Work out the finished part from the listing and answer in its coordinate system (mm). A direction names the side the tool comes from. Round coordinates to 2 decimals unless told otherwise and drop trailing zeros. Order: outer loops, then holes, each group sorted by start corner. A loop starts at its lowest first (then second) coordinate and runs counter-clockwise, first axis right, second up. Notation, with made-up numbers: (38, -35) - (87, -35) arc R14 cw to (87, -30) - close; hole circle Ø2 at (24, 59). An arc over 180 degrees is marked (long way). One line per question, with ' | ' between items. Start each with the question number.
Autodesk Fusion 360 part; units mm, degrees
sketch "Sketch1" plane through (0, 0, 0) normal (0, 0, 1) x (1, 0, 0)
  line L0 (0, 0) -> (80, 0)
  line L1 (80, 0) -> (80, 140)
  line L2 (80, 140) -> (0, 140)
  line L3 (0, 140) -> (0, 0)
  line L4 (40, 140) -> (40, 0) construction
  circle A0 centre (40, 45) radius 7.5
  line L5 (5, 5) -> (75, 5) construction
  line L6 (75, 5) -> (75, 135) construction
  line L7 (75, 135) -> (5, 135) construction
  line L8 (5, 135) -> (5, 5) construction
  circle A1 centre (75, 135) radius 1.65
  circle A2 centre (5, 135) radius 1.65
  circle A3 centre (75, 5) radius 1.65
  circle A4 centre (5, 5) radius 1.65
  circle A5 centre (75, 5) radius 3.15
  circle A6 centre (5, 5) radius 3.15
  circle A7 centre (5, 135) radius 3.15
  circle A8 centre (75, 135) radius 3.65
  circle A9 centre (40, 70) radius 2.5
  dimension "d1" = 80
  dimension "d2" = 140
  dimension "d3" = 15
  dimension "d13" = -5
  dimension "d14" = 3.3
  dimension "d15" = 3.3
  dimension "d16" = 3.3
  dimension "d17" = 3.3
  dimension "d18" = 1.5
  dimension "d19" = 1.5
  dimension "d20" = 1.5
  dimension "d21" = 2
  dimension "d38" = 45
  dimension "d40" = 5
  dimension "d41" = 25
extrude "Extrude1" add sketch "Sketch1" along normal blind 48 contours L0 L1 L2 L3 | A0 | A1 | A2 | A3 | A4 | A5 | A6 | A7 | A8 | A9
shell "Shell1" thickness 3 removed faces 1 at (26.6667, 46.6667, 0)
extrude "Footswitch hole" cut sketch "Sketch1" along normal up to surface (48 mm away) contours A0 | A9
sketch "Sketch3" plane through (0, 0, 0) normal (-1, 0, 0) x (0, -1, 0)
  line L0 (-140, 0) -> (0, 0)
  line L1 (0, 0) -> (0, 48)
  line L2 (0, 48) -> (-140, 48)
  line L3 (-140, 48) -> (-140, 0)
  line L4 (-130, 32) -> (0, 32) construction
  circle A0 centre (-25, 32) radius 7.5
  dimension "d28" = 15
  dimension "d37" = 25
  dimension "d39" = 16
extrude "Extrude5" cut sketch "Sketch3" against normal up to surface (80 mm away) contours A0
fillet "Fillet1" radius 4 8 edges at (0, 0, 24) (3, 3, 22.5) (80, 0, 24) (77, 3, 22.5) (0, 140, 24) (3, 137, 22.5) (77, 137, 22.5) (80, 140, 24)
fillet "Fillets" radius 4 8 edges at (1.1716, 1.1716, 48) (40, 0, 48) (78.8284, 1.1716, 48) (80, 70, 48) (78.8284, 138.8284, 48) (40, 140, 48) (1.1716, 138.8284, 48) (0, 70, 48)
extrude "Extrude3" add sketch "Sketch1" along normal up to surface (45 mm away) contours A5 | A6 | A7 | A8
extrude "Extrude4" cut sketch "Sketch1" along normal up to surface (45 mm away) contours A1 | A2 | A3 | A4
fillet "Fillet3" radius 3 8 edges at (72.5664, 3, 22.5) (77, 7.4336, 22.5) (3, 7.4336, 22.5) (7.4336, 3, 22.5) (7.4336, 137, 22.5) (3, 132.5664, 22.5) (77, 131.9467, 22.5) (71.9467, 137, 22.5)
sketch "Sketch4" plane through (0, 140, 0) normal (0, 1, 0) x (-1, 0, 0)
  line L0 (-4, 44) -> (-76, 44)
  line L1 (-76, 44) -> (-76, 0)
  line L2 (-76, 0) -> (-4, 0)
  line L3 (-4, 0) -> (-4, 44)
  line L4 (-30, 18.7772) -> (-50, 18.7772)
  line L5 (-50, 18.7772) -> (-50, 5.7772)
  line L6 (-50, 5.7772) -> (-30, 5.7772)
  line L7 (-30, 5.7772) -> (-30, 18.7772)
  line L8 (-40, 44) -> (-40, 0) construction
  line L9 (-30, 12.2772) -> (-65, 12.2772) construction
  circle A0 centre (-65, 12.2772) radius 2.5
  dimension "d31" = 20
  dimension "d32" = 13
  dimension "d42" = 5
  dimension "d43" = 15
extrude "Extrude6" cut sketch "Sketch4" against normal up to surface (3 mm away) contours L4 L5 L6 L7 | A0
equation "d38 = 35 mm + 10 mm"
1) Section C-C on y = 25 is taken. Give the vertices of the cut face in (x, z).
2) Straight lines are drawn through the part: line 1 (Y direction, x = 20.5, z = 17.5); line 2 (X direction, y = 77.5, z = 33.5); line 3 (Z direction, x = 30.5, y = 18). For each, find the intervals that lie inside material, in ascending order.
3) Determine the mould class of faces 1 (the cylindrical face through (9.15, 3.694, 22.185)), 2 (the flat face through (47, 71, 48)), 3 (the cylindrical face through (1.203, 69.076, 46.859)), 4 (the cylindrical face through (70.358, 136.295, 22.185)) for opening direction X: released by +X, released by -X, zero draft, split by the parting line, or undercut.
4) For faces 5 (the cylindrical face through (7.208, 7.247, 22.185)), 6 (the cylindrical face through (78.797, 70.924, 46.859)), 7 (the cylindrical face through (62.7, 138.5, 11.3)), determine the directions among +Z, -Z, +X, -X, +Y, -Y from which every point of the face is accessible in a straight line to the end or side of a thin tool.
5) Section D-D on z = 16.5 is taken. Give the number of separate pieces and of enclosed holes in the cut face, and give its area (3 significant figures).
6) Section B-B on y = 70 is taken. Give the vertices of the cut face in (x, z).
7) Flat-ended cylindrical pins translate along their axes: pin 1 (5 mm diameter, centred on x = 12, y = 98.5, fed in from -Z); pin 2 (3 mm diameter, centred on x = 65, z = 12.28, fed in from -Y); pin 3 (1.5 mm diameter, centred on x = 36, y = 139, fed in from +Z); pin 4 (2.5 mm diameter, centred on y = 138.5, z = 12.5, fed in from +X). Find the tip coordinate at first contact, or state that the pin passes through.
8) Section A-A on x = 65 is taken. Give the vertices of the cut face in (y, z).
Recorded:
1) outline: (0, 0) - (3, 0) - (3, 24.5) - (0, 24.5) - close; (0, 39.5) - (3, 39.5) - (3, 45) - (77, 45) - (77, 39.5) - (80, 39.5) - (80, 44) arc R4 ccw to (76, 48) - (4, 48) arc R4 ccw to (0, 44) - close; (77, 0) - (80, 0) - (80, 24.5) - (77, 24.5) - close
2) line 1: y = 0 to 3, 137 to 140 | line 2: x = 0 to 3, 77 to 80 | line 3: z = 45 to 48
3) face 1: undercut | face 2: zero draft | face 3: released by -X | face 4: undercut
4) face 5: -Z | face 6: +Z, +X, +Y, -Y | face 7: +Y
5) separate pieces: 1 | enclosed holes: 4 | area: 1,290 mm²
6) outline: (0, 0) - (3, 0) - (3, 45) - (37.5, 45) - (37.5, 48) - (4, 48) arc R4 ccw to (0, 44) - close; (42.5, 45) - (77, 45) - (77, 0) - (80, 0) - (80, 44) arc R4 ccw to (76, 48) - (42.5, 48) - close
7) pin 1: stops at z = 45 | pin 2: stops at y = 0 | pin 3: stops at z = 47.31 | pin 4: stops at x = 79.8
8) outline: (0, 0) - (3, 0) - (3, 45) - (137, 45) - (137, 14.78) - (140, 14.78) - (140, 44) arc R4 ccw to (136, 48) - (4, 48) arc R4 ccw to (0, 44) - close; (137, 0) - (140, 0) - (140, 9.78) - (137, 9.78) - close
